Can you work these out from the model? Positions are in its coordinate system, mm. Round coordinates to 2 decimals unless told otherwise and drop trailing zeros. Loops run counter-clockwise (first coordinate to the right, second up) from the corner with the lowest first, then second, coordinate; pieces in that order, holes last. Notation, with made-up numbers: M 53.5,50 L 85.5,50 A13 cw 85.5,57 Z; hole C 4.25,-30.5 d2. An arc over 180 degrees is marked long. Use a Markdown table: item, result. Add a question column.
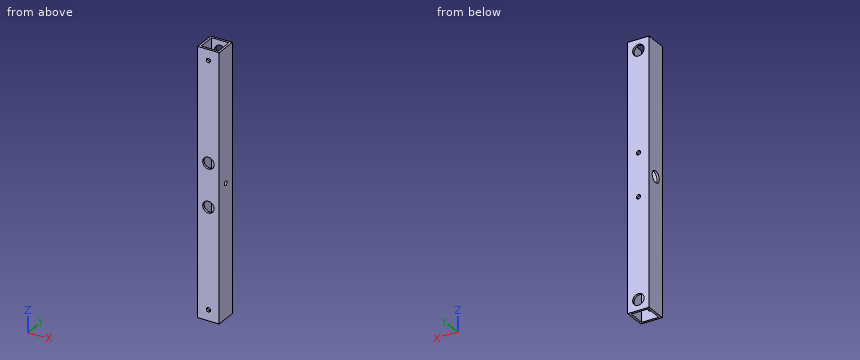
```python
from build123d import *

# Parameters (mm, degrees)
SKETCH_1_W           = 15
SKETCH_1_H           = 15
SKETCH_1_W_2         = 12
SKETCH_1_H_2         = 12
EXTRUDE_2_DEPTH      = 185
SKETCH_2_R           = 4
CUT_EXTRUDE_1_DEPTH  = 10
SKETCH_3_R           = 4
CUT_EXTRUDE_2_DEPTH  = 10
SKETCH_4_R           = 1.5
CUT_EXTRUDE_3_DEPTH  = 10
SKETCH_5_R           = 1.5
CUT_EXTRUDE_4_DEPTH  = 10
SKETCH_6_R           = 1.5
CUT_EXTRUDE_5_DEPTH  = 10
SKETCH_8_R           = 1.5
CUT_EXTRUDE_6_DEPTH  = 10
CUT_EXTRUDE_7_DEPTH  = 10
SKETCH_10_R          = 4
CUT_EXTRUDE_8_DEPTH  = 10
SKETCH_11_R          = 1.5
CUT_EXTRUDE_9_DEPTH  = 10
SKETCH_12_R          = 4
CUT_EXTRUDE_10_DEPTH = 10


with BuildPart() as part:
    # ｽｹｯﾁ1 → ﾎﾞｽ - 押し出し2 (new body)
    with BuildSketch(Plane.XY):
        with Locations((0.489915859, 0.232626086)):
            Rectangle(SKETCH_1_W, SKETCH_1_H)
        with Locations((0.489915859, 0.232626086)):
            Rectangle(SKETCH_1_W_2, SKETCH_1_H_2, mode=Mode.SUBTRACT)
    extrude(amount=EXTRUDE_2_DEPTH)

    # ｽｹｯﾁ2 → ｶｯﾄ - 押し出し1 (cut)
    with BuildSketch(Plane(origin=(0, 7.732626086, 0), x_dir=(1, 0, 0), z_dir=(0, 1, 0))):
        with Locations((0.489915859, -7.5)):
            Circle(SKETCH_2_R)
    extrude(amount=-CUT_EXTRUDE_1_DEPTH, mode=Mode.SUBTRACT)

    # ｽｹｯﾁ3 → ｶｯﾄ - 押し出し2 (cut)
    with BuildSketch(Plane(origin=(0, 7.732626086, 0), x_dir=(1, 0, 0), z_dir=(0, 1, 0))):
        with Locations((0.489915859, -177.5)):
            Circle(SKETCH_3_R)
    extrude(amount=-CUT_EXTRUDE_2_DEPTH, mode=Mode.SUBTRACT)

    # ｽｹｯﾁ4 → ｶｯﾄ - 押し出し3 (cut)
    with BuildSketch(Plane.XZ.offset(7.267373914)):
        with Locations((0.489915859, 7.5)):
            Circle(SKETCH_4_R)
    extrude(amount=-CUT_EXTRUDE_3_DEPTH, mode=Mode.SUBTRACT)

    # ｽｹｯﾁ5 → ｶｯﾄ - 押し出し4 (cut)
    with BuildSketch(Plane.XZ.offset(7.267373914)):
        with Locations((0.489915859, 177.5)):
            Circle(SKETCH_5_R)
    extrude(amount=-CUT_EXTRUDE_4_DEPTH, mode=Mode.SUBTRACT)

    # ｽｹｯﾁ6 → ｶｯﾄ - 押し出し5 (cut)
    with BuildSketch(Plane(origin=(0, 7.732626086, 0), x_dir=(1, 0, 0), z_dir=(0, 1, 0))):
        with Locations((0.489915859, -77.5)):
            Circle(SKETCH_6_R)
    extrude(amount=-CUT_EXTRUDE_5_DEPTH, mode=Mode.SUBTRACT)

    # ｽｹｯﾁ8 → ｶｯﾄ - 押し出し6 (cut)
    with BuildSketch(Plane(origin=(0, 7.732626086, 0), x_dir=(1, 0, 0), z_dir=(0, 1, 0))):
        with Locations((0.489915859, -107.5)):
            Circle(SKETCH_8_R)
    extrude(amount=-CUT_EXTRUDE_6_DEPTH, mode=Mode.SUBTRACT)

    # ｽｹｯﾁ9 → ｶｯﾄ - 押し出し7 (cut)
    with BuildSketch(Plane.XZ.offset(7.267373914)):
        with BuildLine():
            ThreePointArc((4.489915859, 77.5), (3.318342984, 80.328427125), (0.489915859, 81.5))
            Line((0.489915859, 81.5), (0.489915859, 77.5))
            Line((0.489915859, 77.5), (4.489915859, 77.5))
        make_face()
        with BuildLine():
            Line((0.489915859, 77.5), (0.489915859, 81.5))
            ThreePointArc((0.489915859, 81.5), (-2.338511265, 74.671572875), (4.489915859, 77.5))
            Line((4.489915859, 77.5), (0.489915859, 77.5))
        make_face()
    extrude(amount=-CUT_EXTRUDE_7_DEPTH, mode=Mode.SUBTRACT)

    # ｽｹｯﾁ10 → ｶｯﾄ - 押し出し8 (cut)
    with BuildSketch(Plane.XZ.offset(7.267373914)):
        with Locations((0.489915859, 107.5)):
            Circle(SKETCH_10_R)
    extrude(amount=-CUT_EXTRUDE_8_DEPTH, mode=Mode.SUBTRACT)

    # ｽｹｯﾁ11 → ｶｯﾄ - 押し出し9 (cut)
    with BuildSketch(Plane(origin=(7.989915859, 0, 0), x_dir=(0, 0, -1), z_dir=(1, 0, 0))):
        with Locations((-92.5, 0.232626086)):
            Circle(SKETCH_11_R)
    extrude(amount=-CUT_EXTRUDE_9_DEPTH, mode=Mode.SUBTRACT)

    # ｽｹｯﾁ12 → ｶｯﾄ - 押し出し10 (cut)
    with BuildSketch(Plane.ZY.offset(7.010084141)):
        with Locations((92.5, 0.232626086)):
            Circle(SKETCH_12_R)
    extrude(amount=-CUT_EXTRUDE_10_DEPTH, mode=Mode.SUBTRACT)


solid = part.part
```
(1) I'm going to push flat-ended pins straight in: pin 1 (5 mm diameter, centred on x = 6, y = -5, fed in from -Z); pin 2 (6.5 mm diameter, centred on x = 0.49, z = 177.5, fed in from +Y); pin 3 (5 mm diameter, centred on x = 0.49, z = 107.5, fed in from -Y); pin 4 (5 mm diameter, centred on y = 0.23, z = 92.5, fed in from -X). Where does each tip first touch, or does it pass through?
(2) Suppose I cut it at A-A on z = 7.5. List the corners of the cut face in (x, y) for me, and give its area (3 significant figures).
(3) Suppose I cut it at B-B on z = 67. List the corners of the cut face in (x, y) for me, and give its area (3 significant figures).
(4) If I drill on probe 1 along X at (y, z) = (5, 94); probe 2 along X at (y, z) = (6.9, 7.5); probe 3 along Y at (x, z) = (7.05, 92.5), over which ranges is the centre line in solid material (lowest first)? Write a range as [from, to].
Results below:
| question | item | result |
|---|---|---|
| 1 | pin 1 | stops at z = 0 |
| 1 | pin 2 | stops at y = -5.77 |
| 1 | pin 3 | stops at y = 6.23 |
| 1 | pin 4 | stops at x = 6.49 |
| 2 | outline | M -7.01,-7.27 L -1.01,-7.27 L -1.01,-5.77 L -5.51,-5.77 L -5.51,6.23 L -3.51,6.23 L -3.51,7.73 L -7.01,7.73 Z; M 1.99,-7.27 L 7.99,-7.27 L 7.99,7.73 L 4.49,7.73 L 4.49,6.23 L 6.49,6.23 L 6.49,-5.77 L 1.99,-5.77 Z |
| 2 | area | 64.5 mm² |
| 3 | outline | M -7.01,-7.27 L 7.99,-7.27 L 7.99,7.73 L -7.01,7.73 Z; hole M -5.51,-5.77 L 6.49,-5.77 L 6.49,6.23 L -5.51,6.23 Z |
| 3 | area | 81.0 mm² |
| 4 | probe 1 | x = [-7.01, -5.51], [6.49, 7.99] |
| 4 | probe 2 | x = [-7.01, -3.51], [4.49, 7.99] |
| 4 | probe 3 | y = [-7.27, -1.27], [1.73, 7.73] |
